Can you work these out from the model? Positions are in its coordinate system, mm. Face numbers are marked on the shaded views. A direction names the side the tool comes from. Give positions to 0.01 mm unless a question says otherwise; leave off trailing zeros. Loops run counter-clockwise (first coordinate to the right, second up) from the corner with the lowest first, then second, coordinate; pieces in that order, holes last. Notation, with made-up numbers: (4, -17.75) -> (17, -17.75) arc R13 ccw to (17, -4.75) -> close; hole circle Ø8 at (-4.75, -17.75). An arc over 180 degrees is marked (long way). Use CSV: the item, a comma, the result in double quotes.
from build123d import *

# Parameters (mm, degrees)
SKETCH1_W           = 1
SKETCH1_H           = 1
BOSS_EXTRUDE1_DEPTH = 0.5
SKETCH2_W           = 1.5
SKETCH2_H           = 1.5
BOSS_EXTRUDE2_DEPTH = 0.25
SKETCH3_R           = 0.5
BOSS_EXTRUDE3_DEPTH = 0.25
SCALE1_SCALE        = 6


with BuildPart() as part:
    # Sketch1 → Boss-Extrude1 (new body)
    with BuildSketch(Plane(origin=(0, 0, 0), x_dir=(1, 0, 0), z_dir=(0, 1, 0))):
        Rectangle(SKETCH1_W, SKETCH1_H)
    extrude(amount=BOSS_EXTRUDE1_DEPTH)

    # Sketch2 → Boss-Extrude2 (add)
    with BuildSketch(Plane(origin=(0, 0.5, 0), x_dir=(1, 0, 0), z_dir=(0, 1, 0))):
        Rectangle(SKETCH2_W, SKETCH2_H)
    extrude(amount=BOSS_EXTRUDE2_DEPTH)

    # Sketch3 → Boss-Extrude3 (add)
    with BuildSketch(Plane.XZ):
        with Locations(Location((0, 0, 0), (0, 0, 270))):
            Circle(SKETCH3_R)
    extrude(amount=BOSS_EXTRUDE3_DEPTH)


with BuildPart() as part_1:
    # Scale1: scaled about (0, 0.359072941, 0)
    add(part.part.scale(SCALE1_SCALE).moved(Location((0, -1.795364705, 0))))


solid = part_1.part
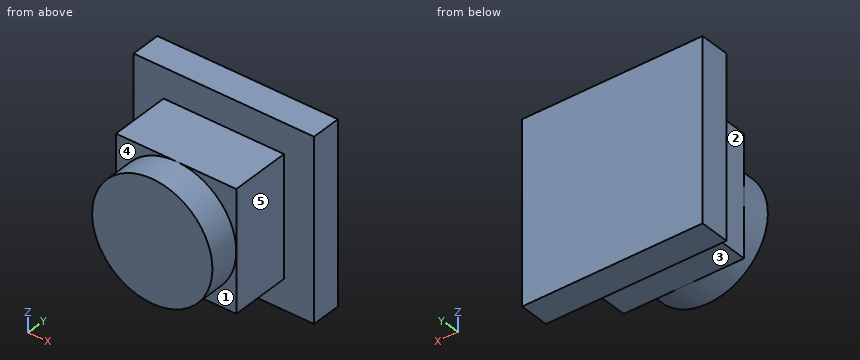
(1) If we section it at D-D, the plane x = 3.25: Write out the boundary of the cut face in (y, z), then the cut area to 3 significant figures.
Answer sheet:
outline,"(1.2, -4.5) -> (2.7, -4.5) -> (2.7, 4.5) -> (1.2, 4.5) -> close"
area,"13.5 mm2"
(2) If I drill on L1, parallel to Y at x = 4, z = 3.75; L2, parallel to X at y = 0.95, z = -2.5, over which ranges is the centre line in solid material (lowest first)? Write a range as from..to.
Answer sheet:
L1,"y = 1.2..2.7"
L2,"x = -3..3"
(3) If we section it at B-B, the plane z = 2.5: Write out the boundary of the cut face in (x, y), then the cut area to 3 significant figures.
Answer sheet:
outline,"(-4.5, 1.2) -> (-3, 1.2) -> (-3, -1.8) -> (-1.66, -1.8) -> (-1.66, -3.3) -> (1.66, -3.3) -> (1.66, -1.8) -> (3, -1.8) -> (3, 1.2) -> (4.5, 1.2) -> (4.5, 2.7) -> (-4.5, 2.7) -> close"
area,"36.5 mm2"
(4) If we section it at C-C, the plane y = -0.35: Write out the boundary of the cut face in (x, z).
Answer sheet:
outline,"(-3, -3) -> (3, -3) -> (3, 3) -> (-3, 3) -> close"
(5) Will these pins go through, and if not, where does the flat tip stop? pin 1 Ø1.5 at (y, z) = (-0.5, 1.5) entering from +X; pin 2 Ø0.9 at (y, z) = (0, 1) entering from -X; pin 3 Ø1.5 at (x, y) = (-0.5, -2.5) entering from -Z.
Answer sheet:
pin 1,"stops at x = 3"
pin 2,"stops at x = -3"
pin 3,"stops at z = -3"
(6) If we section it at A-A, the plane x = 1.5: Write out the boundary of the cut face in (y, z), then the cut area to 3 significant figures.
Answer sheet:
outline,"(-3.3, -2.6) -> (-1.8, -2.6) -> (-1.8, -3) -> (1.2, -3) -> (1.2, -4.5) -> (2.7, -4.5) -> (2.7, 4.5) -> (1.2, 4.5) -> (1.2, 3) -> (-1.8, 3) -> (-1.8, 2.6) -> (-3.3, 2.6) -> close"
area,"39.3 mm2"
(7) Which directions (+Z, -Z, +X, -X, +Y, -Y) give clear straight access to the entire face, cutting with the end or side of a thin tool? Please do the marked faces 1, 2, 3, 4 and 5.
Answer sheet:
face 1,"-Z, +X, -Y"
face 2,"+Z, -Z, -X, -Y"
face 3,"-Z, +X, -X, -Y"
face 4,"+Z, -X, -Y"
face 5,"+Z, -Z, +X, -Y"
